Part model, mm, in its own coordinate system. Face numbers are marked on the shaded views. A direction names the side the tool comes from. Give positions to 0.01 mm unless a question says otherwise; leave off trailing zeros. Order: outer loops, then holes, each group sorted by start corner. A loop starts at its lowest first (then second) coordinate and runs counter-clockwise, first axis right, second up. Notation, with made-up numbers: (28.25, 55.25) - (85.25, 55.25) arc R29 ccw to (85.25, 84.25) - close; hole circle Ø3 at (53, 35). An arc over 180 degrees is marked (long way). One line per item, written item: value.
Autodesk Inventor part; units mm, degrees
ref_plane "YZ Plane" through (0, 0, 0) normal (1, 0, 0) x (0, 1, 0)
ref_plane "XZ Plane" through (0, 0, 0) normal (0, 1, 0) x (-1, 0, 0)
ref_plane "XY Plane" through (0, 0, 0) normal (0, 0, 1) x (1, 0, 0)
sketch "Sketch1" plane through (0, 0, 0) normal (0, 0, 1) x (1, 0, 0)
  line L0 (-30, 30) -> (30, 30)
  line L1 (30, 30) -> (30, -30)
  line L2 (30, -30) -> (-30, -30)
  line L3 (-30, -30) -> (-30, 30)
  line L4 (-30, 30) -> (30, -30) construction
  line L5 (30, 30) -> (-30, -30) construction
  line L6 (0, 0) -> (0, -32.9158)
  circle A0 centre (-12.5, 6.5) radius 1.75
  circle A1 centre (12.5, 6.5) radius 1.75
  line L7 (-8.1, 10.5) -> (8.1, 10.5)
  line L8 (8.1, 10.5) -> (8.1, 2.5)
  line L9 (8.1, 2.5) -> (-8.1, 2.5)
  line L10 (-8.1, 2.5) -> (-8.1, 10.5)
  line L11 (-8.1, 10.5) -> (8.1, 2.5) construction
  line L12 (8.1, 10.5) -> (-8.1, 2.5) construction
  line L13 (13.1, -2.65) -> (-13.1, -2.65)
  line L14 (-13.1, -2.65) -> (-13.1, -22.85)
  line L15 (-13.1, -22.85) -> (13.1, -22.85)
  line L16 (13.1, -22.85) -> (13.1, -2.65)
  line L17 (13.1, -2.65) -> (-13.1, -22.85) construction
  line L18 (-13.1, -2.65) -> (13.1, -22.85) construction
  line L19 (8.9501, 0.5324) -> (10, 12.5324)
  line L20 (-8.9501, 0.5324) -> (-10, 12.5324)
  line L21 (10, 12.5324) -> (-10, 12.5324)
  line L22 (-8.9501, 0.5324) -> (8.9501, 0.5324)
  line L23 (10, 12.5324) -> (-8.9501, 0.5324)
  line L24 (-10, 12.5324) -> (8.9501, 0.5324)
  line L25 (13.1, -16.75) -> (15.6, -16.75)
  line L26 (15.6, -16.75) -> (15.6, -8.75)
  line L27 (15.6, -8.75) -> (13.1, -8.75)
  line L28 (13.1, -8.75) -> (13.1, -16.75)
  line L29 (-13.1, -8.75) -> (-15.6, -8.75)
  line L30 (-15.6, -8.75) -> (-15.6, -16.75)
  line L31 (-15.6, -16.75) -> (-13.1, -16.75)
  line L32 (-13.1, -16.75) -> (-13.1, -8.75)
  line L33 (0, -12.75) -> (7.7881, -12.75)
  point P0 (0, 6.5)
  point P1 (0, 6.2)
  dimension "d0" = 60
  dimension "d1" = 60
  dimension "d10" = 3.5
  dimension "d11" = 3.5
  dimension "d12" = 25
  dimension "d15" = 16.2
  dimension "d16" = 8
  dimension "d21" = 26.2
  dimension "d22" = 20.2
  dimension "d32" = 17.25
  dimension "d33" = 19.25
  dimension "d61" = 5
  dimension "d62" = 20
  dimension "d63" = 12
  dimension "d67" = 0.3
  dimension "d68" = 2.5
  dimension "d69" = 8
extrude "Extrusion1" add sketch "Sketch1" along normal blind 10 contours L0 L1 L2 L3 | L10 L9 L23 L20 L24 L7 | L24 L21 L23 L7 | L23 L19 L24 L9 L8 L7 | L9 L24 L22 L23
extrude "Extrusion10" cut sketch "Sketch1" along normal blind 5 contours L10 L9 L23 L20 L24 L7 | L24 L21 L23 L7 | L23 L19 L24 L9 L8 L7 | L9 L24 L22 L23
fillet "Fillet1" radius 1 4 edges at (10, 12.5324, 2.5) (-10, 12.5324, 2.5) (-8.9501, 0.5324, 2.5) (8.9501, 0.5324, 2.5)
sketch "Sketch2" plane through (0, 0, 0) normal (0, 0, -1) x (-1, 0, 0)
  line L0 (-15.75, -0.5) -> (15.75, -0.5)
  line L1 (15.75, -0.5) -> (15.75, -25)
  line L2 (15.75, -25) -> (-15.75, -25)
  line L3 (-15.75, -25) -> (-15.75, -0.5)
  line L4 (-15.75, -0.5) -> (15.75, -25) construction
  line L5 (15.75, -0.5) -> (-15.75, -25) construction
  line L6 (13.1, -22.85) -> (13.1, -2.65)
  point P0 (0, 0)
  point P1 (0, -12.75)
  point P2 (-15.75, -12.75)
  point P3 (13.1, -12.75)
  dimension "d17" = 31.5
  dimension "d18" = 24.5
extrude "Extrusion2" cut sketch "Sketch2" against normal blind 3.1
sketch "Sketch3" plane through (0, 0, 0) normal (0, 0, -1) x (-1, 0, 0)
  line L0 (-15.5, 13.1) -> (15.5, 13.1)
  line L1 (15.5, 13.1) -> (15.5, -0.1)
  line L2 (15.5, -0.1) -> (-15.5, -0.1)
  line L3 (-15.5, -0.1) -> (-15.5, 13.1)
  line L4 (-15.5, 13.1) -> (15.5, -0.1) construction
  line L5 (15.5, 13.1) -> (-15.5, -0.1) construction
  circle A0 centre (-12.5, 6.5) radius 1.75
  point P0 (0, 0)
  point P1 (0, 6.5)
  dimension "d23" = 31
  dimension "d24" = 13.2
extrude "Extrusion3" cut sketch "Sketch3" against normal blind 1.1 contours L0 L1 L2 L3 | A0
sketch "Sketch4" plane through (0, 0, 0) normal (0, 0, -1) x (-1, 0, 0)
  circle A0 centre (-12.5, 6.5) radius 1.75
  line L0 (-9.65, 8.1454) -> (-9.65, 4.8546)
  line L1 (-9.65, 4.8546) -> (-12.5, 3.2091)
  line L2 (-12.5, 3.2091) -> (-15.35, 4.8546)
  line L3 (-15.35, 4.8546) -> (-15.35, 8.1454)
  line L4 (-15.35, 8.1454) -> (-12.5, 9.7909)
  line L5 (-12.5, 9.7909) -> (-9.65, 8.1454)
  circle A1 centre (12.5, 6.5) radius 1.75
  line L6 (12.5, 9.7909) -> (15.35, 8.1454)
  line L7 (15.35, 8.1454) -> (15.35, 4.8546)
  line L8 (15.35, 4.8546) -> (12.5, 3.2091)
  line L9 (12.5, 3.2091) -> (9.65, 4.8546)
  line L10 (9.65, 4.8546) -> (9.65, 8.1454)
  line L11 (9.65, 8.1454) -> (12.5, 9.7909)
  point P0 (0, 0)
  point P1 (-9.65, 6.5)
  point P2 (-15.35, 6.5)
  dimension "d27" = 5.7
  dimension "d30" = 5.7
extrude "Extrusion4" cut sketch "Sketch4" against normal blind 3.6 contours A0 | L0 L1 L2 L3 L4 L5 | A1 | L6 L7 L8 L9 L10 L11
sketch "Sketch5" plane through (0, 0, 10) normal (0, 0, 1) x (1, 0, 0)
  circle A0 centre (-20, 20) radius 2.85
  line L0 (0, 0) -> (0, 27.5529)
  line L1 (0, 0) -> (35.0302, 0)
  circle A1 centre (20, 20) radius 2.85
  circle A2 centre (-20, -20) radius 2.85
  circle A3 centre (20, -20) radius 2.85
  dimension "d34" = 5.7
  dimension "d35" = 40
  dimension "d36" = 40
extrude "Extrusion5" cut sketch "Sketch5" against normal blind 4
sketch "Sketch6" plane through (0, 0, 0) normal (0, 0, -1) x (-1, 0, 0)
  circle A0 centre (-10, 18) radius 3.9
  circle A1 centre (10, 18) radius 3.9
  line L0 (30, -30) -> (-30, -30)
  line L1 (0, 0) -> (0, 19.7)
  dimension "d39" = 7.8
  dimension "d40" = 7.8
  dimension "d41" = 48
  dimension "d42" = 20
extrude "Extrusion6" cut sketch "Sketch6" against normal through all
sketch "Sketch8" plane through (0, 0, 10) normal (0, 0, 1) x (1, 0, 0)
  line L0 (-13.9, 30) -> (-6.1, 30)
  line L1 (-6.1, 30) -> (-6.1, 13.8)
  line L2 (-6.1, 13.8) -> (-13.9, 13.8)
  line L3 (-13.9, 13.8) -> (-13.9, 30)
  line L4 (0, 0) -> (0, 35.6896)
  line L5 (13.9, 30) -> (6.1, 30)
  line L6 (6.1, 30) -> (6.1, 13.8)
  line L7 (6.1, 13.8) -> (13.9, 13.8)
  line L8 (13.9, 13.8) -> (13.9, 30)
  circle A0 centre (-10, 18) radius 3.9
  line L9 (-10, 18) -> (-10, 21.5524)
  line L10 (30, 30) -> (-30, 30)
  dimension "d46" = 7.8
  dimension "d48" = 4.2
extrude "Extrusion7" cut sketch "Sketch8" against normal blind 5 contours L5 L8 L7 L6 | L0 L1 A0 L3 | A0 L1 L2 L3
sketch "Sketch9" plane through (-20, 20, 6) normal (0, 0, 1) x (1, 0, 0)
  circle A0 centre (0, 0) radius 1.75
  circle A1 centre (40, 0) radius 2.85
  circle A2 centre (40, 0) radius 1.75
  circle A3 centre (0, -40) radius 2.85
  circle A4 centre (0, -40) radius 1.75
  circle A5 centre (40, -40) radius 2.85
  circle A6 centre (40, -40) radius 1.75
  point P0 (20, -20)
  dimension "d51" = 3.5
  dimension "d52" = 3.5
  dimension "d53" = 3.5
  dimension "d54" = 3.5
extrude "Extrusion8" cut sketch "Sketch9" against normal through all contours A0 | A2 | A4 | A6
sketch "Sketch10" plane through (0, 0, 10) normal (0, 0, 1) x (1, 0, 0)
  line L0 (-30, 30) -> (-30, -30)
  line L1 (-20, 10) -> (-30, 10)
  line L2 (-30, 10) -> (-30, -10)
  line L3 (-30, -10) -> (-20, -10)
  line L4 (-20, -10) -> (-20, 10)
  line L5 (-20, 10) -> (-30, -10) construction
  line L6 (-30, 10) -> (-20, -10) construction
  line L7 (0, 0) -> (0, 15.7555)
  line L8 (20, 10) -> (30, 10)
  line L9 (30, 10) -> (30, -10)
  line L10 (30, -10) -> (20, -10)
  line L11 (20, -10) -> (20, 10)
  line L12 (20, 10) -> (30, -10) construction
  line L13 (30, 10) -> (20, -10) construction
  point P0 (-25, 0)
  point P1 (25, 0)
  dimension "d57" = 20
  dimension "d58" = 10
extrude "Extrusion9" cut sketch "Sketch10" against normal blind 5
equation "\"d10\" = d2"
equation "\"d11\" = d2"
equation "\"d30\" = d27"
equation "\"d39\" = d40"
equation "\"d52\" = d51"
equation "\"d53\" = d51"
equation "\"d54\" = d51"
properties part number "power_signal_socket_fixed"
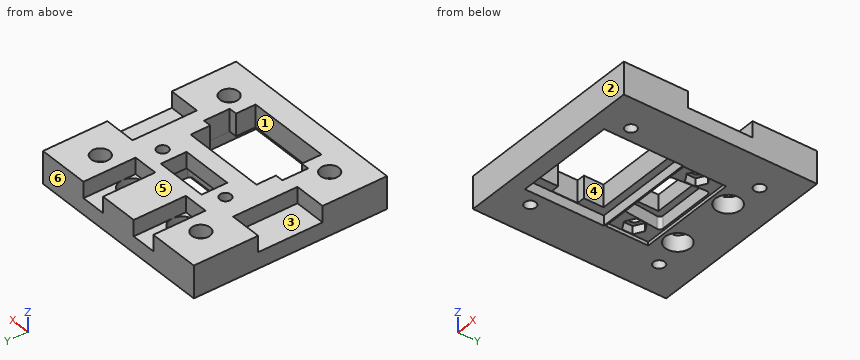
1) Slice it at B-B on x = 19. Write the cut outline in (y, z).
Answer:
outline: (-30, 0) - (-21.44, 0) - (-21.44, 6) - (-22.67, 6) - (-22.67, 10) - (-30, 10) - close; (-18.56, 0) - (18.56, 0) - (18.56, 6) - (17.33, 6) - (17.33, 10) - (-17.33, 10) - (-17.33, 6) - (-18.56, 6) - close; (21.44, 0) - (30, 0) - (30, 10) - (22.67, 10) - (22.67, 6) - (21.44, 6) - close
2) Drop flat-ended pins along their axis: P1, Ø7, axis at x = 10, y = 18, coming from the +Z side; P2, Ø1.5, axis at y = 5.5, z = 7, coming from the +X side. Give the stop position or say it passes through.
Answer:
P1: passes through
P2: stops at x = 20
3) Two-plate mould, pull along Y, no slides. Class the marked faces 4, 5 and 6: pulls with the +Y half, pulls with the -Y half, needs draft (parallel to the pull), parting line crosses it, or undercut.
Answer:
face 4: undercut
face 5: needs draft
face 6: pulls with the +Y half
4) Slice it at C-C on y = 25.5. Write the cut outline in (x, z).
Answer:
outline: (-30, 0) - (30, 0) - (30, 10) - (13.9, 10) - (13.9, 5) - (6.1, 5) - (6.1, 10) - (-6.1, 10) - (-6.1, 5) - (-13.9, 5) - (-13.9, 10) - (-30, 10) - close
5) Wall check: line 1 along X through (y, z) = (6.5, 7.5); line 2 along Y through (x, z) = (7, 8.75); line 3 along X through (y, z) = (26, 5.25). Give the ranges that are in metal, low to high. Write a range as [from, to].
Answer:
line 1: x = [-20, -14.25], [-10.75, -8.1], [8.1, 10.75], [14.25, 20]
line 2: y = [-30, -22.85], [-2.65, 2.5], [10.5, 13.8]
line 3: x = [-30, -13.9], [-6.1, 6.1], [13.9, 30]
6) Which spindle directions (+Z, -Z, +X, -X, +Y, -Y) get a long thin tool onto all of the face, cutting with end or side? Do the marked faces 1, 2 and 3. Say none if no direction does.
Answer:
face 1: +Z, -Z
face 2: +Z, -Z, +X, -X, -Y
face 3: +Z, -X
7) Slice it at A-A on y = -6.5. Write the cut outline in (x, z), then the cut area to 3 significant figures.
Answer:
outline: (-30, 0) - (-15.75, 0) - (-15.75, 3.1) - (-13.1, 3.1) - (-13.1, 10) - (-20, 10) - (-20, 5) - (-30, 5) - close; (13.1, 3.1) - (15.75, 3.1) - (15.75, 0) - (30, 0) - (30, 5) - (20, 5) - (20, 10) - (13.1, 10) - close
area: 222 mm2
8) Slice it at D-D on x = -24. Write the cut outline in (y, z).
Answer:
outline: (-30, 0) - (30, 0) - (30, 10) - (10, 10) - (10, 5) - (-10, 5) - (-10, 10) - (-30, 10) - close
